```python
from build123d import *

# Parameters (mm, degrees)
SKETCH1_R           = 2.5
BOSS_EXTRUDE1_DEPTH = 9.5
BOSS_EXTRUDE2_START = 9
BOSS_EXTRUDE2_DEPTH = 9


with BuildPart() as part:
    # Sketch1 → Boss-Extrude1 (new, symmetric)
    with BuildSketch(Plane(origin=(0, 0, 0), x_dir=(0, 0, -1), z_dir=(1, 0, 0))):
        Circle(SKETCH1_R)
    extrude(amount=BOSS_EXTRUDE1_DEPTH, both=True)

    # Sketch2 → Boss-Extrude2 (add)
    with BuildSketch(Plane(origin=(9.5, 0, 0), x_dir=(0, 0, -1), z_dir=(1, 0, 0)).offset(BOSS_EXTRUDE2_START)):
        with BuildLine():
            Line((-2, 1.5), (-2, -1.5))
            ThreePointArc((-2, -1.5), (0, -2.5), (2, -1.5))
            Line((2, -1.5), (2, 1.5))
            ThreePointArc((2, 1.5), (0, 2.5), (-2, 1.5))
        make_face()
    boss_extrude2 = extrude(amount=-BOSS_EXTRUDE2_DEPTH)

    # Mirror1: Boss-Extrude2 across plane
    add(boss_extrude2.mirror(Plane(origin=(0, 0, 0), x_dir=(0, 0, 1), z_dir=(1, 0, 0))))


solid = part.part
```
Can you work these out from the model? Positions are in its coordinate system, mm. A direction names the side the tool comes from. Round coordinates to 2 decimals unless told otherwise and drop trailing zeros. Loops run counter-clockwise (first coordinate to the right, second up) from the corner with the lowest first, then second, coordinate; pieces in that order, holes last. Notation, with made-up numbers: M 8.25,9.25 L 20.25,9.25 A32 ccw 20.25,43.25 Z; hole C 36,51.25 d5. An arc over 180 degrees is marked long. Answer as a JSON object with one key per item and string values. Group by question number.
Q1. Imagine slicing it at B-B, the plane x = 7. Please give me the cut outline in (y, z), then the cut area to 3 significant figures.
Q2. Please list where these lines run through material, in increasing order: L1, parallel to Z at x = 15.5, y = -0.1; L2, parallel to Y at x = -11, z = -0.2; L3, parallel to X at y = 0.7, z = 2.2.
Q3. Imagine slicing it at A-A, the plane y = 0. Please give me the cut outline in (x, z).
Q4. Will these pins go through, and if not, where does the flat tip stop? pin 1 (1.5 mm diameter, centred on x = 12, y = 0, fed in from +Z); pin 2 (2.5 mm diameter, centred on x = 15.5, y = 0.5, fed in from -Z); pin 3 (1.5 mm diameter, centred on x = 9, y = 1, fed in from -Z).
Q5. Imagine slicing it at D-D, the plane y = -2. Please give me the cut outline in (x, z), then the cut area to 3 significant figures.
Q6. On a 3-axis mill with a long thin cutter (end or side, diameter ignored), from which of +Z, -Z, +X, -X, +Y, -Y can I reach the whole of each face in a straight line? I mean faces 1 (the flat face through (14, 0, -2)), 2 (the flat face through (-14, 0, -2)), 3 (the flat face through (14, 0, 2)). Say none if no direction works.
Q7. Imagine slicing it at C-C, the plane z = -1.45. Please give me the cut outline in (x, y), then the cut area to 3 significant figures.
Findings:
{
 "1": {"outline": "C 0,0 d5", "area": "19.6 mm2"},
 "2": {"L1": "z = -2 to 2", "L2": "y = -2.49 to 2.49", "L3": "x = -9.5 to 9.5"},
 "3": {"outline": "M -18.5,-2 L -9.5,-2 L -9.5,-2.5 L 9.5,-2.5 L 9.5,-2 L 18.5,-2 L 18.5,2 L 9.5,2 L 9.5,2.5 L -9.5,2.5 L -9.5,2 L -18.5,2 Z"},
 "4": {"pin 1": "stops at z = 2", "pin 2": "stops at z = -2", "pin 3": "stops at z = -2.49"},
 "5": {"outline": "M -18.5,-1.5 L 18.5,-1.5 L 18.5,1.5 L -18.5,1.5 Z", "area": "111 mm2"},
 "6": {"face 1": "-Z, +X, +Y, -Y", "face 2": "-Z, -X, +Y, -Y", "face 3": "+Z, +X, +Y, -Y"},
 "7": {"outline": "M -18.5,-2.04 L 18.5,-2.04 L 18.5,2.04 L -18.5,2.04 Z", "area": "151 mm2"}
}
